Read the model definition and answer for the solid it produces. Units are mm, in the model's axes. A direction names the side the tool comes from. Round coordinates to 2 decimals unless told otherwise and drop trailing zeros. Write each loop counter-clockwise with the first axis right and the second up, starting at its lowest first coordinate (ties: lowest second). Pieces come first, ordered by that corner, then holes. Notation, with made-up numbers: M -19.5,26 L 22.5,26 A11 ccw 22.5,42 Z; hole C 34.25,-14.5 d4. An arc over 180 degrees is marked long. Use one line per item in the form item = value. Start each with the question number.
```python
from build123d import *

# Parameters (mm, degrees)
CROQUIS1_W                 = 7
CROQUIS1_H                 = 10.8
SALIENTE_EXTRUIR1_DEPTH    = 17.5
CROQUIS4_W                 = 3.5
CROQUIS4_H                 = 14.5
CORTAR_EXTRUIR1_DEPTH      = 17.5
CORTAR_EXTRUIR2_DEPTH      = 22.723029255
CORTAR_EXTRUIR2_DEPTH_BACK = 22.723029255
CROQUIS6_W                 = 4
CROQUIS6_H                 = 14.5
CORTAR_EXTRUIR3_DEPTH      = 17.5


with BuildPart() as part:
    # Croquis1 → Saliente-Extruir1 (new body)
    with BuildSketch(Plane.XY):
        with Locations((3.5, 5.4)):
            Rectangle(CROQUIS1_W, CROQUIS1_H)
    extrude(amount=SALIENTE_EXTRUIR1_DEPTH)

    # Croquis4 → Cortar-Extruir1 (cut)
    with BuildSketch(Plane(origin=(0, 10.8, 0), x_dir=(1, 0, 0), z_dir=(0, 1, 0))):
        with Locations((3.25, -8.75)):
            Rectangle(CROQUIS4_W, CROQUIS4_H)
    extrude(amount=-CORTAR_EXTRUIR1_DEPTH, mode=Mode.SUBTRACT)

    # Croquis5 → Cortar-Extruir2 (cut, two sides: drawn at the far end of the back side and taken through both)
    with BuildSketch(Plane(origin=(7, 0, 0), x_dir=(0, 0, -1), z_dir=(1, 0, 0)).offset(-CORTAR_EXTRUIR2_DEPTH_BACK)):
        with BuildLine():
            Line((-7.903521509, 5.161580042), (-4, 10.8))
            Line((-4, 10.8), (-17.5, 10.8))
            Line((-17.5, 10.8), (-17.5, 4.3))
            Line((-17.5, 4.3), (-9.547905892, 4.3))
            ThreePointArc((-9.547905892, 4.3), (-8.619692532, 4.528441376), (-7.903521509, 5.161580042))
        make_face()
    extrude(amount=CORTAR_EXTRUIR2_DEPTH + CORTAR_EXTRUIR2_DEPTH_BACK, mode=Mode.SUBTRACT)

    # Croquis6 → Cortar-Extruir3 (cut)
    with BuildSketch(Plane(origin=(0, 10.8, 0), x_dir=(1, 0, 0), z_dir=(0, 1, 0))):
        with Locations((3.5, -8.75)):
            Rectangle(CROQUIS6_W, CROQUIS6_H)
    extrude(amount=-CORTAR_EXTRUIR3_DEPTH, mode=Mode.SUBTRACT)


solid = part.part
```
Q1. Each of these flat-tipped pins is pushed along its axis until it touches: pin 1 Ø1.2 at (x, y) = (3.5, 7.5) entering from +Z; pin 2 Ø3.5 at (x, z) = (4.5, 13) entering from +Y; pin 3 Ø4 at (y, z) = (6.5, 15.5) entering from +X. Where does it stop, or does it pass through?
Q2. Find section C-C on y = 2. Write down the section's boundary in (x, z).
Q3. Find section D-D on x = 6.5. Write down the section's boundary in (y, z), and give its area (3 significant figures).
Q4. A tool of negligible diameter and unlimited length cuts with its end or side. For faces 4 (the face through (3, 5, 1.5)), 5 (the face through (3.5, 4.3, 16.2)), 6 (the face through (0, 4, 7)), from which of +Z, -Z, +X, -X, +Y, -Y can it reach the whole face along a straight path? Write none if from no direction.
Q5. Straight lines are drawn through the part: line 1 (X direction, y = 1.5, z = 4); line 2 (Z direction, x = 5.25, y = 3.25); line 3 (Z direction, x = 2, y = 9.5). For each, find the intervals that lie inside material, in ascending order. Write a range as [from, to].
Q6. For a pull along Z with two mould halves and no side action, classify faces 1 (the face through (1.5, 4, 7)), 2 (the face through (3, 10.8, 1)), 3 (the face through (0.74, 7.94, 5.98)) as +Z half, -Z half, draft (parallel to the pull), parting line (faces both ways), or undercut.
Q7. Find section A-A on x = 2.75. Write down the section's boundary in (y, z).
Q8. Find section B-B on z = 13.75. Write down the section's boundary in (x, y), and give its area (3 significant figures).
Response:
q1.pin_1 = 1.5
q1.pin_2 = 4.3
q1.pin_3 = through
q2.outline = M 0,0 L 7,0 L 7,17.5 L 0,17.5 Z; hole M 1.5,1.5 L 5.5,1.5 L 5.5,16 L 1.5,16 Z
q3.outline = M 0,0 L 10.8,0 L 10.8,4 L 5.16,7.9 A2 cw 4.3,9.55 L 4.3,17.5 L 0,17.5 Z
q3.area = 116 mm²
q4.face_4 = +Y, -Y
q4.face_5 = +Z, +X, -X, +Y
q4.face_6 = +Z, -Z, -X, +Y, -Y
q5.line_1 = [0, 1.5], [5.5, 7]
q5.line_2 = [0, 1.5], [16, 17.5]
q5.line_3 = [0, 1.5]
q6.face_1 = undercut
q6.face_2 = draft
q6.face_3 = +Z half
q7.outline = M 0,0 L 10.8,0 L 10.8,1.5 L 0,1.5 Z; M 0,16 L 4.3,16 L 4.3,17.5 L 0,17.5 Z
q8.outline = M 0,0 L 1.5,0 L 1.5,4.3 L 0,4.3 Z; M 5.5,0 L 7,0 L 7,4.3 L 5.5,4.3 Z
q8.area = 12.9 mm²
